Part model, mm, in its own coordinate system. A direction names the side the tool comes from. Give positions to 0.01 mm unless a question says otherwise; leave off trailing zeros. Write each loop counter-clockwise with the first axis right and the second up, starting at its lowest first coordinate (ties: lowest second). Pieces come first, ordered by that corner, then holes.
from build123d import *

# Parameters (mm, degrees)
F0_W     = 12
F0_H     = 12
F1_DEPTH = 10
F0_W_2   = 2
F0_H_2   = 3.1217085198
F0_R     = 1.4457822704
F2_DEPTH = 6
F0_R_2   = 4
F0_W_3   = 25
F0_H_3   = 0.9
F3_DEPTH = 2
F5_DEPTH = 12
F6_R     = 2
F7_R     = 1
F8_W     = 18
F8_H     = 1.9928832203
F9_DEPTH = 25


# Not quite as in the source:
# - a feature names something its author has since deleted; it is built from what else it names


with BuildPart() as f1:
    # F0 (on Top) → F1 (new body)
    with BuildSketch(Plane.XY):
        Polygon((15, -15), (15, 15), (-15, 15), (-15, 6), (-15, -6), (-15, -15), align=None)
        Polygon((12.5, 13.4), (13.4, 13.4), (13.4, -13.4), (-13.4, -13.4), (-13.4, 13.4), (-12.5, 13.4), align=None, mode=Mode.SUBTRACT)
        with Locations((-21, 0)):
            Rectangle(F0_W, F0_H)
    extrude(amount=F1_DEPTH)

    # F0 (on Top) → F2 (join)
    with BuildSketch(Plane.XY):
        Polygon((-9.5, -3.5004718229), (-12.5, -1.4055506326), (-12.5, -12.5), (-7.5, -12.5), (-7.5, -4.8970859498), align=None)
        with Locations((-10.5, -9.9175968207)):
            Rectangle(F0_W_2, F0_H_2, mode=Mode.SUBTRACT)
        with Locations((-10.256325826, -5.7152966037)):
            Circle(F0_R, mode=Mode.SUBTRACT)
        Polygon((-9.5, 6.1722276732), (-12.5, 8.2671488635), (-12.5, -1.4055506326), (-9.5, -3.5004718229), align=None)
        Polygon((12.5, -1.4055506326), (12.5, 8.2671488635), (9.5, 6.1722276732), (9.5, -3.5004718229), align=None)
        Polygon((12.5, -12.5), (12.5, -1.4055506326), (9.5, -3.5004718229), (7.5, -4.8970859498), (7.5, -12.5), align=None)
        with Locations((10.5, -9.9175968207)):
            Rectangle(F0_W_2, F0_H_2, mode=Mode.SUBTRACT)
        with Locations((10.256325826, -5.7152966037)):
            Circle(F0_R, mode=Mode.SUBTRACT)
        Polygon((13.4, -13.4), (13.4, 13.4), (12.5, 13.4), (12.5, 12.5), (12.5, 8.2671488635), (12.5, -1.4055506326), (12.5, -12.5), (7.5, -12.5), (-7.5, -12.5), (-12.5, -12.5), (-12.5, -1.4055506326), (-12.5, 8.2671488635), (-12.5, 12.5), (-12.5, 13.4), (-13.4, 13.4), (-13.4, -13.4), align=None)
    extrude(amount=F2_DEPTH)

    # F0 (on Top) → F3 (join)
    with BuildSketch(Plane.XY):
        Polygon((12.5, 8.2671488635), (12.5, 12.5), (-12.5, 12.5), (-12.5, 8.2671488635), (-9.5, 6.1722276732), (-9.5, -3.5004718229), (-7.5, -4.8970859498), (-7.5, -12.5), (7.5, -12.5), (7.5, -4.8970859498), (9.5, -3.5004718229), (9.5, 6.1722276732), align=None)
        with Locations((0, -3.5)):
            Circle(F0_R_2, mode=Mode.SUBTRACT)
        with Locations((10.256325826, -5.7152966037)):
            Circle(F0_R)
        with Locations((10.5, -9.9175968207)):
            Rectangle(F0_W_2, F0_H_2)
        with Locations((-10.5, -9.9175968207)):
            Rectangle(F0_W_2, F0_H_2)
        with Locations((-10.256325826, -5.7152966037)):
            Circle(F0_R)
        with Locations((0, 12.95)):
            Rectangle(F0_W_3, F0_H_3)
    extrude(amount=F3_DEPTH)

    # F4 (on face) → F5 (cut)
    with BuildSketch(Plane(origin=(-27, 0, 0), x_dir=(0, -1, 0), z_dir=(-1, 0, 0))):
        Polygon((-3.6, 5.1207184246), (3.6, 5.1207184246), (0, 8.8730510324), align=None)
        Polygon((0, 1.3683858167), (3.6, 5.1207184246), (-3.6, 5.1207184246), align=None)
    extrude(amount=-F5_DEPTH, mode=Mode.SUBTRACT)

    # F6
    f6_edges = [f1.edges().sort_by_distance(p)[0] for p in [
        (15, 15, 5),
        (-15, 15, 5),
        (-15, -15, 5),
        (15, -15, 5),
    ]]
    fillet(f6_edges, radius=F6_R)

    # F7
    f7_edges = [f1.edges().sort_by_distance(p)[0] for p in [
        (-15, -9.5, 0),
        (0, -15, 0),
    ]]
    fillet(f7_edges, radius=F7_R)

    # F8 (on face) → F9 (cut)
    with BuildSketch(Plane.XZ.offset(15)):
        with Locations((0, 9.0035583898)):
            Rectangle(F8_W, F8_H)
    extrude(amount=-F9_DEPTH, mode=Mode.SUBTRACT)


solid = f1.part
1) Saw through at B-B (x = -17). Write the cut outline in (y, z).
Check result:
outline: (-6, 0) - (6, 0) - (6, 10) - (-6, 10) - close; hole (-3.6, 5.12) - (0, 1.37) - (3.6, 5.12) - (0, 8.87) - close
2) Mould opens along Z. For faces 1 (the flat face through (10, -11.478, 4)), 2 (the flat face through (-21.084, -1.825, 6.971)), 3 (the flat face through (10, -10, 2)) say: +Z half, -Z half, draft (parallel to the pull), parting line (faces both ways), or undercut.
Check result:
face 1: draft
face 2: undercut
face 3: +Z half
3) Drill centre lines: L1, parallel to Y at x = 11, z = 6.25; L2, parallel to Y at x = 0, z = 1.45; L3, parallel to Y at x = -9, z = 5.5. Where is each one in solid material? Low to high.
Check result:
L1: y = -15 to -13.4, 13.4 to 15
L2: y = -15 to -7.5, 0.5 to 15
L3: y = -15 to -6.43, -5 to -3.85, 13.4 to 15
4) Saw through at C-C (z = 9.5). Write the cut outline in (x, y).
Check result:
outline: (-27, -6) - (-15, -6) - (-15, -13) arc R2 ccw to (-13, -15) - (-9, -15) - (-9, -13.4) - (-13.4, -13.4) - (-13.4, 13.4) - (13.4, 13.4) - (13.4, -13.4) - (9, -13.4) - (9, -15) - (13, -15) arc R2 ccw to (15, -13) - (15, 13) arc R2 ccw to (13, 15) - (-13, 15) arc R2 ccw to (-15, 13) - (-15, 6) - (-27, 6) - close
5) Saw through at D-D (x = 8). Write the cut outline in (y, z), and give its area (3 significant figures).
Check result:
outline: (-15, 1) arc R1 ccw to (-14, 0) - (14, 0) arc R1 ccw to (15, 1) - (15, 10) - (13.4, 10) - (13.4, 2) - (-4.55, 2) - (-4.55, 6) - (-13.4, 6) - (-13.4, 8.01) - (-15, 8.01) - close
area: 117 mm2
6) Flat gauge pins, fed straight in: P1, Ø0.8, axis at y = -14.5, z = 8.5, coming from the +X side; P2, Ø3, axis at y = 11, z = 4.5, coming from the -X side; P3, Ø4.5, axis at x = 10.26, y = -5.72, coming from the +Z side. Where does each tip first touch, or does it go through?
Check result:
P1: stops at x = 14.67
P2: stops at x = -15
P3: stops at z = 6
7) 3-axis set-ups, long thin cutter, end or side, ignore diameter. For faces 4 (the flat face through (-10, -6, 2)), 5 (the flat face through (-9, -14, 9)), 6 (the cylindrical face through (-14.699, 9.451, 0.285)), 7 (the flat face through (-15, 10, 5)), 8 (the flat face through (-2.2, 0.2, 0)): which of +Z, -Z, +X, -X, +Y, -Y reach the whole face in a straight line?
Check result:
face 4: +Z
face 5: +Z, -Y
face 6: -Z, -X, +Y
face 7: +Z, -Z, -X, +Y
face 8: -Z, +X, -X, +Y, -Y
8) Saw through at A-A (x = 0). Write the cut outline in (y, z), and give its area (3 significant figures).
Check result:
outline: (-15, 1) arc R1 ccw to (-14, 0) - (-7.5, 0) - (-7.5, 2) - (-12.5, 2) - (-12.5, 6) - (-13.4, 6) - (-13.4, 8.01) - (-15, 8.01) - close; (0.5, 0) - (14, 0) arc R1 ccw to (15, 1) - (15, 10) - (13.4, 10) - (13.4, 2) - (0.5, 2) - close
area: 69.6 mm2
